Geometry: final body of the model. Coordinates: model frame, mm. Give positions to 0.01 mm unless a question says otherwise; leave off trailing zeros. Order: outer loops, then holes, each group sorted by start corner. A loop starts at its lowest first (then second) coordinate and runs counter-clockwise, first axis right, second up. Notation, with made-up numbers: (20, 89.25) - (62, 89.25) arc R26 cw to (62, 128.25) - close; hole circle Ø1 at (7.5, -1). An arc over 180 degrees is marked (long way). Use one line per item in the form item = value.
from build123d import *

# Parameters (mm, degrees)
SKETCH1_W                   = 88.9
SKETCH1_H                   = 101.6
BOSS_EXTRUDE1_DEPTH         = 9.525
F_1_4_0_25_DIAMETER_HOLE1_D = 6.35
F_1_4_0_25_DIAMETER_HOLE2_D = 6.35


with BuildPart() as part:
    # Sketch1 → Boss-Extrude1 (new body)
    with BuildSketch(Plane.XY):
        with Locations((-44.45, 50.8)):
            Rectangle(SKETCH1_W, SKETCH1_H)
    extrude(amount=BOSS_EXTRUDE1_DEPTH)

    # 1/4 (0.25) Diameter Hole1 (through all)
    with Locations(Plane.XY.offset(9.525)):
        with Locations((-35.759581135, 85.220282149), (-41.783720078, 43.051309551)):
            Hole(F_1_4_0_25_DIAMETER_HOLE1_D / 2)

    # 1/4 (0.25) Diameter Hole2 (through all)
    with Locations(Plane.XY.offset(9.525)):
        with Locations((-47.80785902, 85.220282149)):
            Hole(F_1_4_0_25_DIAMETER_HOLE2_D / 2)


solid = part.part
(1) Pull-direction query (Y, two-part tool) for faces 1 (the face through (-45, 0, 5)), 2 (the face through (-45, 52, 9.525)), 3 (the face through (-43.249, 40.235, 4.696)); classes: released by +Y, released by -Y, zero draft, split by the parting line, or undercut.
Computed values:
face_1 = released by -Y
face_2 = zero draft
face_3 = undercut
(2) Contact query for a flat-ended pin moving along its axis: pin 1 Ø3 at (y, z) = (46, 2) entering from +X. Output: stop coordinate, or through.
Computed values:
pin_1 = 0
(3) Ray query, line 1 along Y through (x, z) = (-47.5, 3.25); line 2 along X through (y, z) = (43, 7.75); line 3 along Y through (x, z) = (-41.5, 1). Return the intervals inside material, ascending.
Computed values:
line_1 = 0 to 82.06, 88.38 to 101.6
line_2 = -88.9 to -44.96, -38.61 to 0
line_3 = 0 to 39.89, 46.21 to 101.6
(4) Cut plane A-A on y = 84. Output: boundary loops of the cut face in (x, z) (3 decimals).
Computed values:
outline = (-88.9, 0) - (-50.739, 0) - (-50.739, 9.525) - (-88.9, 9.525) - close; (-44.877, 0) - (-38.691, 0) - (-38.691, 9.525) - (-44.877, 9.525) - close; (-32.828, 0) - (0, 0) - (0, 9.525) - (-32.828, 9.525) - close
